The figure shows three views and two pictorial views of one solid part (mm, origin at its lowest corner). Answer the questions. A direction names the side the tool comes from. Round coordinates to 2 decimals unless told otherwise and drop trailing zeros. Loops run counter-clockwise (first coordinate to the right, second up) from the corner with the lowest first, then second, coordinate; pieces in that order, holes last. Notation, with made-up numbers: (4.5, 73.25) -> (30.5, 73.25) arc R24 ccw to (30.5, 100.25) -> close; hole circle Ø9 at (7.5, 10.25). An arc over 180 degrees is marked (long way). Use a Markdown table: item, result. Add a question column.
Q1. Consider line 1 (Y direction, x = 60, z = 7); line 2 (Y direction, x = 94.5, z = 27.5); line 3 (Z direction, x = 89.5, y = 9). Determine where each line is inside the solid, lowest interval first.
Q2. Section D-D on x = 28 is taken. Give the vertices of the cut face in (y, z).
Q3. Section C-C on y = 76.5 is taken. Give the vertices of the cut face in (x, z), then the cut area to 3 significant figures.
Q4. Section A-A on y = 40 is taken. Give the vertices of the cut face in (x, z), then the cut area to 3 significant figures.
Q5. Which of the six approach directions +Z, -Z, +X, -X, +Y, -Y give full straight-line access (tool end or side, diameter ignored) to the marked faces 4, 5, 6, 7 and 8?
Q6. Section B-B on x = 60 is taken. Give the vertices of the cut face in (y, z).
Q7. For a pull along Y with two mould halves and no side action, classify the marked faces 1, 2 and 3 as released by +Y, released by -Y, zero draft, split by the parting line, or undercut.
Q8. Given pin 1 Ø10 at (x, z) = (14, 68) entering from -Y; pin 2 Ø12.5 at (y, z) = (21, 23) entering from +X; pin 3 Ø1.5 at (x, y) = (27.5, 36.5) entering from +Z; pin 4 Ø2 at (y, z) = (80, 14.5) entering from -X, each flat-ended and moving along its own axis, determine where each tip first touches the part or whether it passes through.
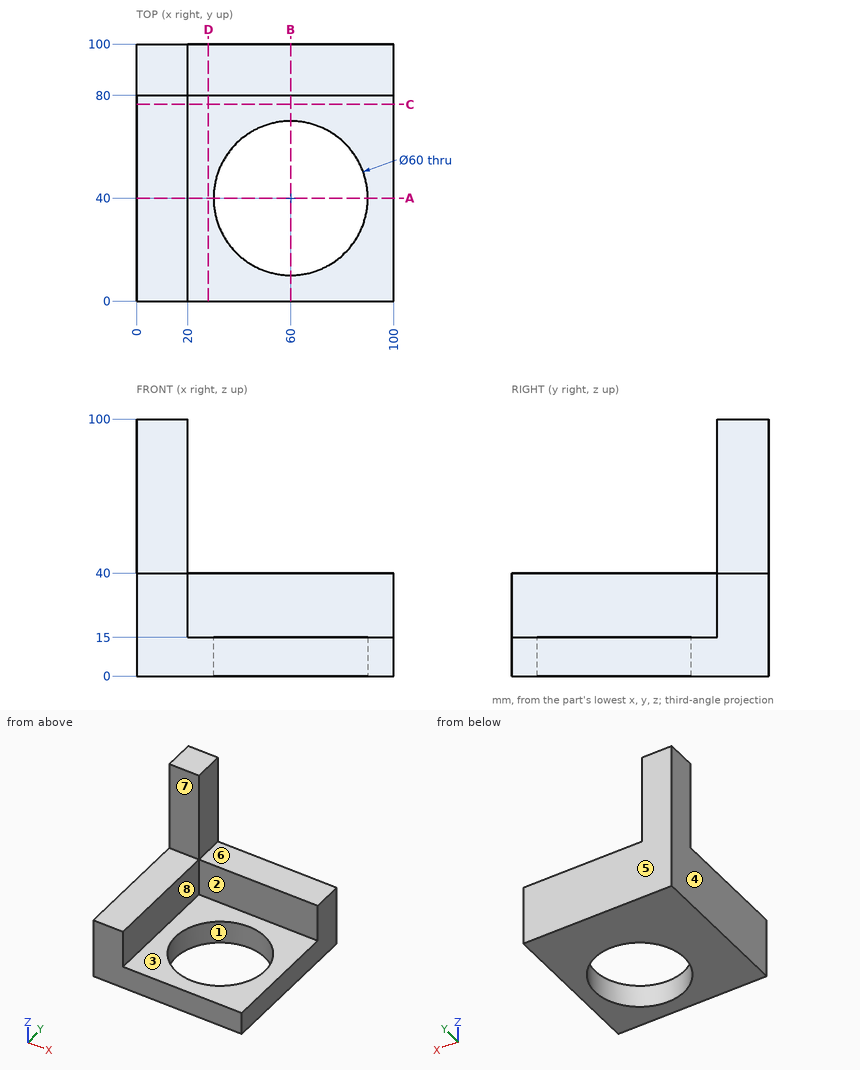
Checked values:
| question | item | result |
|---|---|---|
| 1 | line 1 | y = 0 to 10, 70 to 100 |
| 1 | line 2 | y = 80 to 100 |
| 1 | line 3 | z = 0 to 15 |
| 2 | outline | (0, 0) -> (100, 0) -> (100, 40) -> (80, 40) -> (80, 15) -> (0, 15) -> close |
| 3 | outline | (0, 0) -> (100, 0) -> (100, 15) -> (20, 15) -> (20, 40) -> (0, 40) -> close |
| 3 | area | 2,000 mm2 |
| 4 | outline | (0, 0) -> (30, 0) -> (30, 15) -> (20, 15) -> (20, 40) -> (0, 40) -> close; (90, 0) -> (100, 0) -> (100, 15) -> (90, 15) -> close |
| 4 | area | 1,100 mm2 |
| 5 | face 4 | +Z, -Z, -X, +Y, -Y |
| 5 | face 5 | +Z, -Z, +X, -X, +Y |
| 5 | face 6 | +Z, +X, +Y, -Y |
| 5 | face 7 | +Z, +X, -X, -Y |
| 5 | face 8 | +Z, +X, -Y |
| 6 | outline | (0, 0) -> (10, 0) -> (10, 15) -> (0, 15) -> close; (70, 0) -> (100, 0) -> (100, 40) -> (80, 40) -> (80, 15) -> (70, 15) -> close |
| 7 | face 1 | undercut |
| 7 | face 2 | released by -Y |
| 7 | face 3 | zero draft |
| 8 | pin 1 | stops at y = 80 |
| 8 | pin 2 | stops at x = 20 |
| 8 | pin 3 | stops at z = 15 |
| 8 | pin 4 | stops at x = 0 |
